Geometry check sheet. Reference: the model listing, model coordinates, mm. Face numbers are marked on the shaded views. A direction names the side the tool comes from. Round coordinates to 2 decimals unless told otherwise and drop trailing zeros. Order: outer loops, then holes, each group sorted by start corner. A loop starts at its lowest first (then second) coordinate and runs counter-clockwise, first axis right, second up. Notation, with made-up numbers: (8.25, 52.5) - (36.25, 52.5) arc R25 ccw to (36.25, 78.5) - close; hole circle Ø8 at (-0.75, 46). An arc over 180 degrees is marked (long way). Return JSON: item names as keys, results as strings. Group by question number.
Q1. Sectioned sample at D-D, the plane z = 20.5. Record the cut outline in (x, y).
Q2. Gauge pin test, flat ends, axial feed: pin 1 Ø1.5 at (y, z) = (-2, 42.5) entering from -X; pin 2 Ø1.5 at (x, y) = (-27, -11.5) entering from +Z; pin 3 Ø3 at (y, z) = (6.5, 48.5) entering from -X. Record the tip position at first contact, or that the pin passes through.
Q3. Sectioned sample at B-B, the plane y = 8. Record the cut outline in (x, z), then the cut area to 3 significant figures.
Q4. Draft check along Z on the marked faces 1, 2 and 3. Enter one of: pulls with the +Z half, pulls with the -Z half, needs draft (parallel to the pull), parting line crosses it, or undercut.
Q5. Tool access check on the marked faces 4, 5 and 6. Record the directions out of +Z, -Z, +X, -X, +Y, -Y that give a thin tool (end or side, any length) a straight path to the whole face; none if there is none.
Q6. Material ranges on line 1 along Y through (x, z) = (36.5, 70); line 2 along X through (y, z) = (-2, 76); line 3 along Z through (x, y) = (9.5, 18.5), recorded low to high.
Q7. Sectioned sample at A-A, the plane x = -34.5. Record the cut outline in (y, z).
Q8. Sectioned sample at C-C, the plane x = 45. Record the cut outline in (y, z).
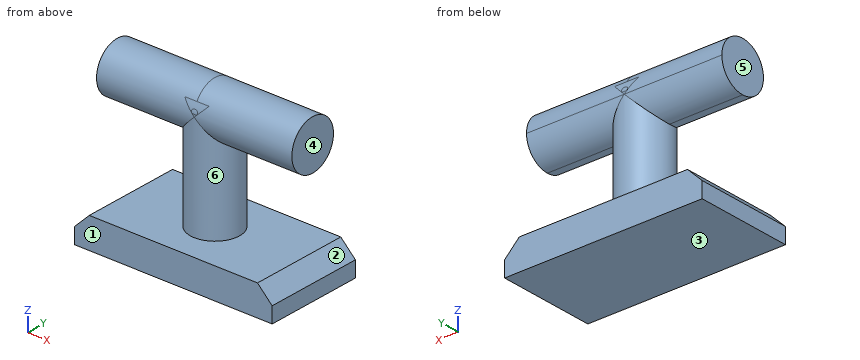
```python
from build123d import *

# Parameters (mm, degrees)
F0_W         = 12.7
F0_H         = 6.35
F0_H_2       = 47.7120632529
F0_H_3       = 15.7879367471
F0_W_2       = 38.6885356486
F2_DEPTH     = 25.4
F4_DEPTH     = 50.8
F5_SIZE      = 7.62
F6_T4_ANGLE  = 174.612014659
F6_S5_R      = 12.7
F6_T6_DEPTH  = 17
F6_T10_ANGLE = 174.612014659
F6_S11_R     = 12.7
F6_T12_DEPTH = 17


# Not quite as in the source:
# - a fillet or chamfer that OpenCascade refuses, or shapes differently, is made with other operations: its cross-section is extruded or revolved along the edge and cut away or added


with BuildPart() as f1:
    # F0 (on Front) → F1 (revolve)
    with BuildSketch(Plane.XZ):
        with Locations((-6.35, 73.025)):
            Rectangle(F0_W, F0_H)
        with Locations((-6.35, 66.675)):
            Rectangle(F0_W, F0_H)
        with Locations((-6.35, 39.6439683735)):
            Rectangle(F0_W, F0_H_2)
    revolve(axis=Axis((0, 0, 38.1), (0, 0, 1)))

    # F0 (on Front) → F2 (join, symmetric)
    with BuildSketch(Plane.XZ):
        with Locations((-6.35, 7.8939683735)):
            Rectangle(F0_W, F0_H_3)
        with Locations((6.35, 7.8939683735)):
            Rectangle(F0_W, F0_H_3)
        with Locations((-32.0442678243, 7.8939683735)):
            Rectangle(F0_W_2, F0_H_3)
        with Locations((32.0442678243, 7.8939683735)):
            Rectangle(F0_W_2, F0_H_3)
    extrude(amount=F2_DEPTH, both=True)

    # F3 (on Right) → F4 (join, symmetric)
    with BuildSketch(Plane.YZ):
        with BuildLine():
            ThreePointArc((0, 57.15), (8.9802561211, 60.8697438789), (12.7, 69.85))
            ThreePointArc((12.7, 69.85), (-8.9802561211, 78.8302561211), (0, 57.15))
        make_face()
    extrude(amount=F4_DEPTH, both=True)

    # F5
    f5_edges = [f1.edges().sort_by_distance(p)[0] for p in [
        (-51.388536, 0, 15.787937),
        (51.388536, 0, 15.787937),
    ]]
    chamfer(f5_edges, length=F5_SIZE)

    # F6: fillet of radius 5.08 on 3 edges, made by hand


with BuildPart() as f6_tool2:
    # F6_s3 → F6_t4 (revolve)
    with BuildSketch(Plane(origin=(0, 0, 0), x_dir=(0, 0, 1), z_dir=(0.0470017192, -0.9988948085, 0))):
        with BuildLine():
            ThreePointArc((71.12, -12.7), (74.7121024484, -11.2121024484), (76.2, -7.62))
            Line((76.2, -7.62), (76.2, -12.7))
            Line((76.2, -12.7), (71.12, -12.7))
        make_face()
    revolve(axis=Axis((0, 0, 76.2), (0, 0, 1)), revolution_arc=F6_T4_ANGLE)

    # F6_s5 → F6_t6 (cut, symmetric)
    with BuildSketch(Plane.YZ):
        with Locations((0, 69.85)):
            Circle(F6_S5_R)
    extrude(amount=F6_T6_DEPTH, both=True, mode=Mode.SUBTRACT)


with BuildPart() as f1_1:
    add(f1.part)

    # F6_t1: cut F6_tool2
    add(f6_tool2.part, mode=Mode.SUBTRACT)


with BuildPart() as f6_tool8:
    # F6_s9 → F6_t10 (revolve)
    with BuildSketch(Plane(origin=(0, 0, 0), x_dir=(0, 0, 1), z_dir=(-0.0470017192, 0.9988948085, 0))):
        with BuildLine():
            ThreePointArc((71.12, -12.7), (74.7121024484, -11.2121024484), (76.2, -7.62))
            Line((76.2, -7.62), (76.2, -12.7))
            Line((76.2, -12.7), (71.12, -12.7))
        make_face()
    revolve(axis=Axis((0, 0, 76.2), (0, 0, 1)), revolution_arc=F6_T10_ANGLE)

    # F6_s11 → F6_t12 (cut, symmetric)
    with BuildSketch(Plane.YZ):
        with Locations((0, 69.85)):
            Circle(F6_S11_R)
    extrude(amount=F6_T12_DEPTH, both=True, mode=Mode.SUBTRACT)


with BuildPart() as f1_2:
    add(f1_1.part)

    # F6_t7: cut F6_tool8
    add(f6_tool8.part, mode=Mode.SUBTRACT)


solid = f1_2.part
```
Reply:
{
 "1": {"outline": "circle Ø25.4 at (0, 0)"},
 "2": {"pin 1": "x = -12.64", "pin 2": "z = 76.61", "pin 3": "x = -11.67"},
 "3": {"outline": "(-51.39, 0) - (51.39, 0) - (51.39, 8.17) - (43.77, 15.79) - (9.86, 15.79) - (9.86, 59.99) - (50.8, 59.99) - (50.8, 79.71) - (-50.8, 79.71) - (-50.8, 59.99) - (-9.86, 59.99) - (-9.86, 15.79) - (-43.77, 15.79) - (-51.39, 8.17) - close", "area": "4,440 mm^2"},
 "4": {"face 1": "needs draft", "face 2": "undercut", "face 3": "pulls with the -Z half"},
 "5": {"face 4": "+Z, +X, +Y, -Y", "face 5": "+Z, -X, +Y, -Y", "face 6": "none"},
 "6": {"line 1": "-12.7 to 12.7", "line 2": "-50.8 to 50.8", "line 3": "0 to 15.79"},
 "7": {"outline": "(-25.4, 0) - (25.4, 0) - (25.4, 15.79) - (-25.4, 15.79) - close; circle Ø25.4 at (0, 69.85)"},
 "8": {"outline": "(-25.4, 0) - (25.4, 0) - (25.4, 14.56) - (-25.4, 14.56) - close; circle Ø25.4 at (0, 69.85)"}
}
